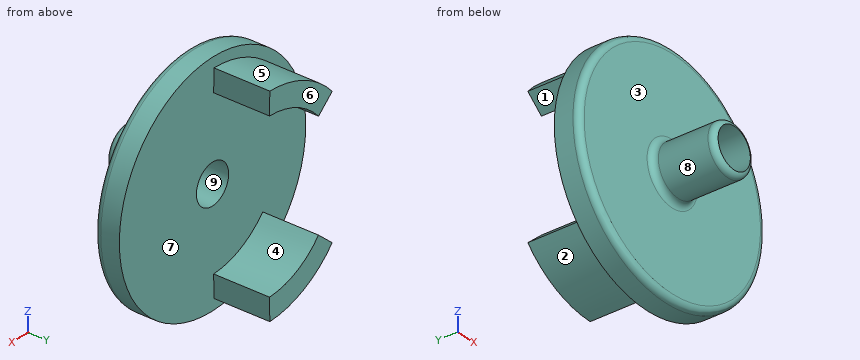
from build123d import *

# Parameters (mm, degrees)
SKETCH1_R           = 18.5
BOSS_EXTRUDE1_DEPTH = 4
SKETCH3_R           = 4
BOSS_EXTRUDE2_DEPTH = 10
FILLET1_R           = 1
FILLET2_R           = 1
BOSS_EXTRUDE3_DEPTH = 9
SKETCH5_R           = 3.2
CUT_EXTRUDE1_DEPTH  = 30.673220359


with BuildPart() as part:
    # Sketch1 → Boss-Extrude1 (new body)
    with BuildSketch(Plane(origin=(0, 0, 0), x_dir=(1, 0, 0), z_dir=(0, 1, 0))):
        with Locations(Location((0, 0, 0), (0, 0, 270))):
            Circle(SKETCH1_R)
    extrude(amount=BOSS_EXTRUDE1_DEPTH)

    # Sketch3 → Boss-Extrude2 (add)
    with BuildSketch(Plane.XZ):
        with Locations(Location((0, 0, 0), (0, 0, 270))):
            Circle(SKETCH3_R)
    extrude(amount=BOSS_EXTRUDE2_DEPTH)

    # Fillet1
    fillet1_edges = [part.edges().sort_by_distance(p)[0] for p in [
        (0, -10, 4),
    ]]
    fillet(fillet1_edges, radius=FILLET1_R)

    # Fillet2
    fillet2_edges = [part.edges().sort_by_distance(p)[0] for p in [
        (0, 0, -18.5),
        (0, 0, 4),
    ]]
    fillet(fillet2_edges, radius=FILLET2_R)

    # Sketch4 → Boss-Extrude3 (add)
    with BuildSketch(Plane(origin=(0, 4, 0), x_dir=(1, 0, 0), z_dir=(0, 1, 0))):
        with BuildLine():
            Line((-12.675055994, 11.02646614), (-9.958972567, 8.663651967))
            ThreePointArc((-9.958972567, 8.663651967), (-5.574490656, 11.965160004), (-0.226257983, 13.198060741))
            Line((-0.226257983, 13.198060741), (-0.287964706, 16.797531852))
            ThreePointArc((-0.287964706, 16.797531852), (-7.094806289, 15.22838546), (-12.675055994, 11.02646614))
        make_face()
        with BuildLine():
            Line((-9.958972567, -8.663651967), (-12.675055994, -11.02646614))
            ThreePointArc((-12.675055994, -11.02646614), (-7.094806289, -15.22838546), (-0.287964706, -16.797531852))
            Line((-0.287964706, -16.797531852), (-0.226257983, -13.198060741))
            ThreePointArc((-0.226257983, -13.198060741), (-5.574490656, -11.965160004), (-9.958972567, -8.663651967))
        make_face()
    extrude(amount=BOSS_EXTRUDE3_DEPTH)

    # Sketch5 → Cut-Extrude1 (cut, through all)
    with BuildSketch(Plane(origin=(0, 4, 0), x_dir=(1, 0, 0), z_dir=(0, 1, 0))):
        with Locations(Location((0, 0, 0), (0, 0, 270))):
            Circle(SKETCH5_R)
    extrude(amount=-CUT_EXTRUDE1_DEPTH, mode=Mode.SUBTRACT)


solid = part.part
The listing builds one solid part. Answer for the finished solid, in the listing's coordinates (mm). Face numbers are marked on the shaded views. A direction names the side the tool comes from. Round coordinates to 2 decimals unless told otherwise and drop trailing zeros. Write each loop counter-clockwise with the first axis right and the second up, starting at its lowest first coordinate (ties: lowest second). Pieces come first, ordered by that corner, then holes. Notation, with made-up numbers: M 68,-24 L 83,-24 A32 ccw 83,15 Z; hole C 81,-35 d8. An arc over 180 degrees is marked long. Write each question's results on one line, items separated by ' | '. Start each with the question number.
Item 1: Which of the six approach directions +Z, -Z, +X, -X, +Y, -Y give full straight-line access (tool end or side, diameter ignored) to the marked faces 1, 2, 3, 4 and 5?
Item 2: Find section C-C on y = -7.75. Write down the section's boundary in (x, z).
Item 3: Given pin 1 Ø10 at (x, z) = (14, -5.5) entering from -Y; pin 2 Ø1.5 at (x, y) = (-11.5, 7) entering from +Z; pin 3 Ø3 at (x, z) = (4, 0) entering from +Y, each flat-ended and moving along its own axis, determine where each tip first touches the part or whether it passes through.
Item 4: Find section A-A on z = 0. Write down the section's boundary in (x, y).
Item 5: Straight lines are drawn through the part: probe 1 along X at (y, z) = (-4.5, 0); probe 2 along Y at (x, z) = (-9.5, 10); probe 3 along Y at (x, z) = (8, 9). For each, find the intervals that lie inside material, in ascending order.
Item 6: Find section B-B on y = 6.5. Write down the section's boundary in (x, z).
Item 7: The mould has two halves that part along Z. Classify the marked faces 6, 7, 8 and 9: +Z half, -Z half, draft (parallel to the pull), parting line (faces both ways), or undercut.
Answer block:
1) face 1: -X, +Y | face 2: -Z, -X, +Y | face 3: -Y | face 4: +X, +Y | face 5: +Z, -X, +Y
2) outline: C 0,0 d8; hole C 0,0 d6.4
3) pin 1: stops at y = 0 | pin 2: stops at z = 12.91 | pin 3: stops at y = 4
4) outline: M -18.5,1 A1 ccw -17.5,0 L -5,0 A1 cw -4,-1 L -4,-9 A1 ccw -3.2,-9.98 L -3.2,4 L -18.5,4 Z; M 3.2,-9.98 A1 ccw 4,-9 L 4,-1 A1 cw 5,0 L 17.5,0 A1 ccw 18.5,1 L 18.5,4 L 3.2,4 Z
5) probe 1: x = -4 to -3.2, 3.2 to 4 | probe 2: y = 0 to 13 | probe 3: y = 0 to 4
6) outline: M -12.68,-11.03 A16.8 ccw -0.29,-16.8 L -0.23,-13.2 A13.2 cw -9.96,-8.66 Z; M -12.68,11.03 L -9.96,8.66 A13.2 cw -0.23,13.2 L -0.29,16.8 A16.8 ccw Z
7) face 6: draft | face 7: undercut | face 8: parting line | face 9: undercut
